from build123d import *

# Parameters (mm, degrees)
F0_R     = 7.5
F1_DEPTH = 25
F2_R     = 2
F3_DEPTH = 5
F7_DEPTH = 3
F11_R    = 2


# Not quite as in the source:
# - a fillet or chamfer that OpenCascade refuses, or shapes differently, is made with other operations: its cross-section is extruded or revolved along the edge and cut away or added


with BuildPart() as f1:
    # F0 (on Top) → F1 (new body)
    with BuildSketch(Plane.XY):
        Circle(F0_R)
    extrude(amount=F1_DEPTH)

    # F2 (on face) → F3 (join)
    with BuildSketch(Plane(origin=(0, 0, 0), x_dir=(1, 0, 0), z_dir=(0, 0, -1))):
        Circle(F2_R)
    extrude(amount=F3_DEPTH)

    # F4 (on face) → F5 (revolve)
    with BuildSketch(Plane(origin=(0, 0, -5), x_dir=(1, 0, 0), z_dir=(0, 0, -1))):
        with BuildLine():
            Line((0, 2), (0, 2.5))
            ThreePointArc((0, 2.5), (-2.5, 0), (0, -2.5))
            Line((0, -2.5), (0, -2))
            ThreePointArc((0, -2), (-2, 0), (0, 2))
        make_face()
        with BuildLine():
            Line((0, -2), (0, 2))
            ThreePointArc((0, 2), (-2, 0), (0, -2))
        make_face()
    revolve(axis=Axis((0, 0, -5), (0, 1, 0)))

    # F6 (on face) → F7 (cut)
    with BuildSketch(Plane.XY.offset(25)):
        with BuildLine():
            add(Edge.make_bspline(
                [(0, 4), (-3.897114317, 4), (-1.9485571585, -2), (0, -8), (1.9485571585, -2), (3.897114317, 4), (0, 4)],
                knots=[0, 0, 0, 2.0943951024, 2.0943951024, 4.1887902048, 4.1887902048, 6.2831853072, 6.2831853072, 6.2831853072], degree=2, weights=[1, 0.5, 1, 0.5, 1, 0.5, 1]))
        make_face()
    extrude(amount=-F7_DEPTH, mode=Mode.SUBTRACT)

    # F8 (on face) → F9 (revolve, cut)
    with BuildSketch(Plane.XY.offset(22)):
        with BuildLine():
            ThreePointArc((1.8, -2.4), (2.683281573, -1.3416407865), (3, 0))
            ThreePointArc((3, 0), (2.683281573, 1.3416407865), (1.8, 2.4))
            add(Edge.make_bspline(
                [(1.8, -2.4), (1.8810311774, -2.2079260981), (1.9485571585, -2), (2.6913429511, 0.2871870789), (1.8, 2.4)],
                knots=[4.0484923357, 4.0484923357, 4.0484923357, 4.1887902048, 4.1887902048, 5.3448576064, 5.3448576064, 5.3448576064], degree=2, weights=[0.9375, 0.9665063509, 1, 0.7240092377, 0.7527020789]))
        make_face()
        with BuildLine():
            Line((0, -3), (0, 3))
            ThreePointArc((0, 3), (-0.9486832981, 2.8460498942), (-1.8, 2.4))
            add(Edge.make_bspline(
                [(-1.8, 2.4), (-2.6913429511, 0.2871870789), (-1.9485571585, -2), (-1.8810311774, -2.2079260981), (-1.8, -2.4)],
                knots=[0.9383277008, 0.9383277008, 0.9383277008, 2.0943951024, 2.0943951024, 2.2346929715, 2.2346929715, 2.2346929715], degree=2, weights=[0.7527020789, 0.7240092377, 1, 0.9665063509, 0.9375]))
            ThreePointArc((-1.8, -2.4), (-0.9486832981, -2.8460498942), (0, -3))
        make_face()
    revolve(axis=Axis((0, 0, 22), (0, -1, 0)), mode=Mode.SUBTRACT)

    # F10: chamfer of 5 x 4 on 1 edges, made by hand

    # F10_s1 → F10_t2 (revolve, cut)
    with BuildSketch(Plane.XZ):
        Polygon((7.5, 21), (2.5, 25), (7.5, 25), align=None)
    revolve(axis=Axis((0, 0, 25), (0, 0, 1)), mode=Mode.SUBTRACT)

    # F11
    f11_edges = [f1.edges().sort_by_distance(p)[0] for p in [
        (-7.5, 0, 0),
    ]]
    fillet(f11_edges, radius=F11_R)


solid = f1.part
Part model, mm, in its own coordinate system. Coordinates: 2 decimals unless noted, no trailing zeros. Loops run counter-clockwise (first coordinate to the right, second up) from the corner with the lowest first, then second, coordinate; pieces in that order, holes last. Notation, with made-up numbers: (-26.5, 50) -> (-21.5, 50) arc R13 ccw to (-21.5, 75) -> close; hole circle Ø8 at (-25.75, 33.25). An arc over 180 degrees is marked (long way). Use a Markdown table: item, result. Add a question column.
Item 1: Pull direction Z, two halves, no side cores. Call faces 1 (the conical face through (-2.74, 0.121, 24.806)), 2 (the cylindrical face through (0, 2, -2)), 3 (the cylindrical face through (-7.493, 0.33, 11.367)): +Z half, -Z half, draft (parallel to the pull), parting line (faces both ways), or undercut.
Item 2: Probe probe 1 along X at (y, z) = (-1.25, 19.5); probe 2 along Z at (x, y) = (2.5, 3.25); probe 3 along X at (y, z) = (-6, 14). List the from-to ranges inside material, lowest first.
Item 3: Band-saw the part on B-B on z = 0.5. Write the cut outline in (x, y).
Item 4: Flat gauge pins, fed straight in: P1, Ø1.8, axis at x = 0.5, y = 3, coming from the +Z side; P2, Ø3, axis at x = 2.5, y = -5.5, coming from the -Z side; P3, Ø1.5, axis at x = 0, y = 3.5, coming from the +Z side; P4, Ø5.5, axis at x = -1.5, y = 2, coming from the -Z side. Where does each tip first touch, or does it go through?
Item 5: Band-saw the part on A-A on z = 13. Write the cut outline in (x, y), plus the area to 3 significant figures.
Geometry says:
| question | item | result |
|---|---|---|
| 1 | face 1 | +Z half |
| 1 | face 2 | undercut |
| 1 | face 3 | draft |
| 2 | probe 1 | -7.4 to -1.09, 1.09 to 7.4 |
| 2 | probe 2 | 0 to 23.72 |
| 2 | probe 3 | -4.5 to 4.5 |
| 3 | outline | circle Ø13.65 at (0, 0) |
| 4 | P1 | z = 24.25 |
| 4 | P2 | z = 0 |
| 4 | P3 | z = 23.9 |
| 4 | P4 | z = -7.5 |
| 5 | outline | circle Ø15 at (0, 0) |
| 5 | area | 177 mm² |
